Verification items for the finished model (mm, model axes). Coordinates: 2 decimals unless noted, no trailing zeros. Loops run counter-clockwise (first coordinate to the right, second up) from the corner with the lowest first, then second, coordinate; pieces in that order, holes last. Notation, with made-up numbers: (46.25, -27) - (54.25, -27) arc R23 cw to (54.25, 11) - close; hole circle Ø4 at (54, 9). An arc over 180 degrees is marked (long way). One line per item, written item: value. Start each with the question number.
(1) Thickness scan on probe 1 along X at (y, z) = (9.7, 22.5); probe 2 along X at (y, z) = (11.7, 49); probe 3 along X at (y, z) = (11.6, 41.5). Record the ranges inside material, lowest first. Write a range as [from, to].
(2) Section check A-A (x = 0). Record the boundary of the cut face in (y, z), plus the area to 3 significant figures.
(3) Gauge pin test, flat ends, axial feed: P1, Ø1, axis at x = 2.5, z = 9.5, coming from the -Y side; P2, Ø1.5, axis at y = 9.5, z = 7.5, coming from the +X side; P3, Ø1.5, axis at x = 2, y = 9.5, coming from the +Z side; P4, Ø1.2, axis at x = -2, z = 28, coming from the -Y side. Record the tip position at first contact, or that the pin passes through.
(4) Section check B-B (x = -2.25). Record the boundary of the cut face in (y, z), plus the area to 3 significant figures.
```python
from build123d import *

# Parameters (mm, degrees)
CYLINDER001_R     = 0.9
CYLINDER001_DEPTH = 55
BOX006_W          = 2.42
BOX006_H          = 1.69
BOX006_DEPTH      = 55
BOX005_W          = 2.42
BOX005_H          = 1.69
BOX005_DEPTH      = 55
EXTRUDE010_DEPTH  = 55
FILLET010_R       = 0.5


with BuildPart() as cilindro:
    # Cylinder001 → Cylinder001 (new body)
    with BuildSketch(Plane(origin=(0, 12.21, 0), x_dir=(1, 0, 0), z_dir=(0, 0, 1))):
        Circle(CYLINDER001_R)
    extrude(amount=CYLINDER001_DEPTH)


with BuildPart() as cubo_der:
    # Box006 → Box006 (new body)
    with BuildSketch(Plane(origin=(1.21, 8.809483, 0), x_dir=(1, 0, 0), z_dir=(0, 0, 1))):
        with Locations((1.21, 0.845)):
            Rectangle(BOX006_W, BOX006_H)
    extrude(amount=BOX006_DEPTH)


with BuildPart() as obj1:
    # Box005 → Box005 (new body)
    with BuildSketch(Plane(origin=(-3.63, 8.809483, 0), x_dir=(1, 0, 0), z_dir=(0, 0, 1))):
        with Locations((1.21, 0.845)):
            Rectangle(BOX005_W, BOX005_H)
    extrude(amount=BOX005_DEPTH)


with BuildPart() as obj2:
    # Sketch009 → Extrude010 (new body)
    with BuildSketch(Plane.XY):
        with BuildLine():
            ThreePointArc((-3.632024, 11.657294), (0, 8.809483), (3.632024, 11.657294))
            ThreePointArc((3.632024, 11.657294), (0, 12.21), (-3.632024, 11.657294))
        make_face()
    extrude(amount=EXTRUDE010_DEPTH)

    # Cut004: cut obj1
    add(obj1.part, mode=Mode.SUBTRACT)

    # Cut005: cut Cubo der
    add(cubo_der.part, mode=Mode.SUBTRACT)

    # Cut006: cut Cilindro
    add(cilindro.part, mode=Mode.SUBTRACT)

    # Fillet010
    fillet010_edges = [obj2.edges().sort_by_distance(p)[0] for p in [
        (-3.128114, 10.499483, 27.5),
        (-3.632024, 11.657294, 27.5),
        (-1.21, 10.499483, 27.5),
        (-0.899389, 12.17683, 27.5),
        (3.128114, 10.499483, 27.5),
        (1.21, 10.499483, 27.5),
        (1.21, 9.010627, 27.5),
        (-1.21, 9.010627, 27.5),
        (0.899389, 12.17683, 27.5),
        (3.632024, 11.657294, 27.5),
    ]]
    fillet(fillet010_edges, radius=FILLET010_R)


solid = obj2.part
```
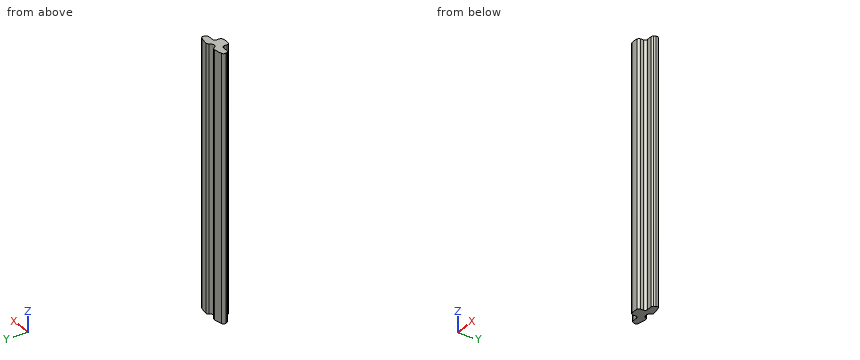
Responses:
1. probe 1: x = [-1.21, 1.21]
1. probe 2: x = [-3.32, -0.74], [0.74, 3.32]
1. probe 3: x = [-3.41, -0.66], [0.66, 3.41]
2. outline: (8.81, 0) - (11.31, 0) - (11.31, 55) - (8.81, 55) - close
2. area: 138 mm²
3. P1: stops at y = 10.5
3. P2: stops at x = 1.28
3. P3: passes through
3. P4: stops at y = 10.39
4. outline: (10.5, 0) - (12, 0) - (12, 55) - (10.5, 55) - close
4. area: 82.6 mm²
